Geometry: see drawing. Coordinates: mm, zero at the bounding-box minimum. Round coordinates to 2 decimals unless told otherwise and drop trailing zeros. Loops run counter-clockwise (first coordinate to the right, second up) from the corner with the lowest first, then second, coordinate; pieces in that order, holes last. Notation, with made-up numbers: M 65.25,11.25 L 117.25,11.25 A24 cw 117.25,42.25 Z; hole C 62,17.5 d10. An arc over 180 degrees is marked long. Answer as a JSON object with one key per item and string values.
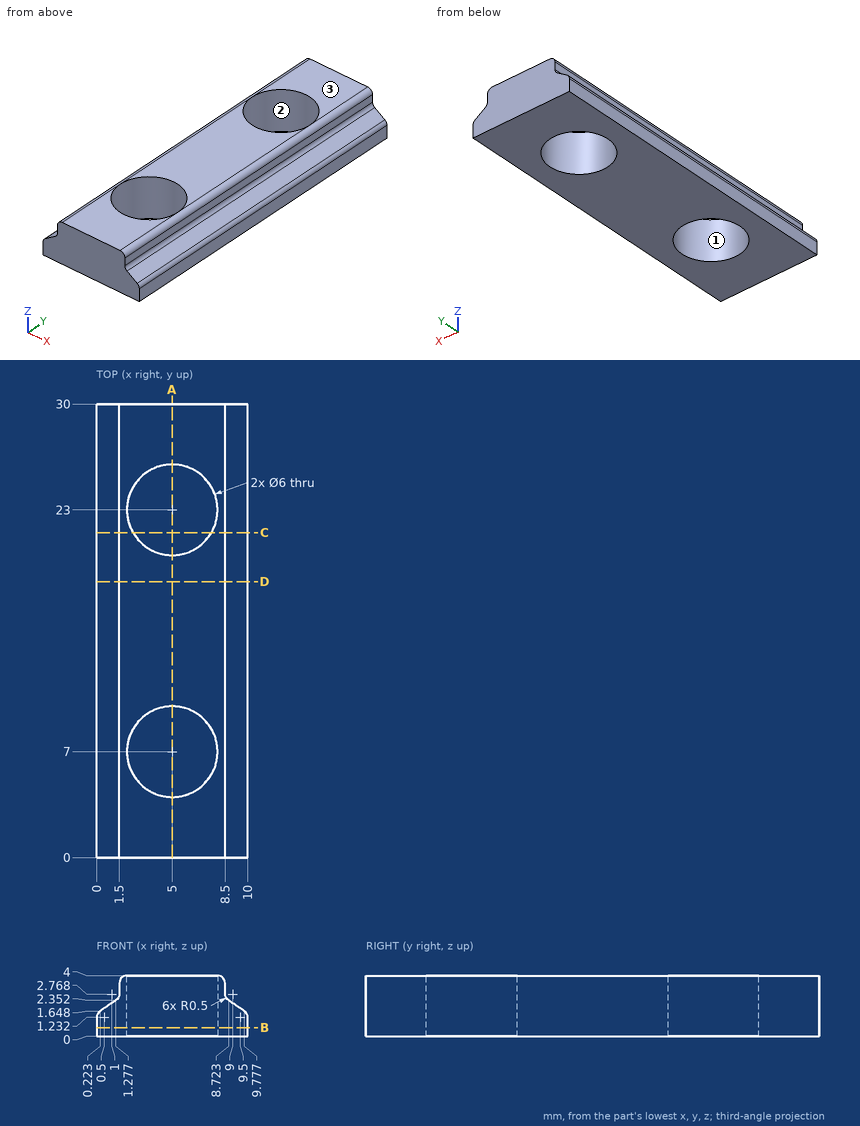
1) Section query B-B (z = 0.55). Return the cut outline in (x, y).
Results:
{"outline": "M 0,0 L 10,0 L 10,30 L 0,30 Z; hole C 5,7 d6; hole C 5,23 d6"}
2) Section query D-D (y = 18.25). Return the cut outline in (x, z).
Results:
{"outline": "M 0,0 L 10,0 L 10,1.23 A0.5 ccw 9.78,1.65 L 8.72,2.35 A0.5 cw 8.5,2.77 L 8.5,3.5 A0.5 ccw 8,4 L 2,4 A0.5 ccw 1.5,3.5 L 1.5,2.77 A0.5 cw 1.28,2.35 L 0.22,1.65 A0.5 ccw 0,1.23 Z"}
3) Section query C-C (y = 21.5). Return the cut outline in (x, z), and give its area (3 significant figures).
Results:
{"outline": "M 0,0 L 2.4,0 L 2.4,4 L 2,4 A0.5 ccw 1.5,3.5 L 1.5,2.77 A0.5 cw 1.28,2.35 L 0.22,1.65 A0.5 ccw 0,1.23 Z; M 7.6,0 L 10,0 L 10,1.23 A0.5 ccw 9.78,1.65 L 8.72,2.35 A0.5 cw 8.5,2.77 L 8.5,3.5 A0.5 ccw 8,4 L 7.6,4 Z", "area": "13.1 mm2"}
4) Pull-direction query (X, two-part tool) for the marked faces 1, 2 and 3; classes: +X half, -X half, draft (parallel to the pull), parting line (faces both ways), or undercut.
Results:
{"face 1": "undercut", "face 2": "undercut", "face 3": "draft"}
5) Pin query (flat end, axial travel): P1, Ø0.6, axis at y = 22, z = 3, coming from the -X side (1 decimal); P2, Ø1, axis at x = 3.5, y = 4.5, coming from the -Z side. Return the tip coordinate at first contact, or that it passes through.
Results:
{"P1": "x = 1.5", "P2": "z = 0"}
6) Ray query, line 1 (Y direction, x = 5, z = 1.2); line 2 (X direction, y = 7, z = 2.35) (1 decimal); line 3 (Y direction, x = 7, z = 1.9) (1 decimal). Return the intervals inside material, ascending.
Results:
{"line 1": "0 to 4, 10 to 20, 26 to 30", "line 2": "1.3 to 2, 8 to 8.7", "line 3": "0 to 4.8, 9.2 to 20.8, 25.2 to 30"}
7) Section query A-A (x = 5). Return the cut outline in (y, z).
Results:
{"outline": "M 0,0 L 4,0 L 4,4 L 0,4 Z; M 10,0 L 20,0 L 20,4 L 10,4 Z; M 26,0 L 30,0 L 30,4 L 26,4 Z"}
